The model under review builds one solid part; all positions refer to its coordinate system, in mm. Face numbers are marked on the shaded views. A direction names the side the tool comes from. Coordinates: 2 decimals unless noted, no trailing zeros. Loops run counter-clockwise (first coordinate to the right, second up) from the corner with the lowest first, then second, coordinate; pieces in that order, holes last. Notation, with made-up numbers: M 4.5,49.25 L 51.5,49.25 A28 cw 51.5,88.25 Z; hole C 5,-35.5 d2. An arc over 180 degrees is marked long. Use one line per item in the form item = value.
```python
from build123d import *

# Parameters (mm, degrees)
F3_W     = 193.8
F3_H     = 30.8805991608
F2_DEPTH = 65.3571831062
F4_R     = 6
F5_DEPTH = 5


with BuildPart() as f1:
    # F0 (on Front) → F1 (revolve)
    with BuildSketch(Plane.XZ):
        Polygon((-44.3082220923, 17.75), (-44.3082220923, 0), (345.4917779077, 0), (345.4917779077, 28), (98.3917779077, 28), (98.3917779077, 43.6), (74.3917779077, 43.6), (74.3917779077, 28), (-15.4082220923, 28), (-15.4082220923, 17.75), align=None)
    revolve(axis=Axis((24.5496360249, 0, 0), (1, 0, 0)))

    # F3 (on Front) → F2 (cut, symmetric)
    with BuildSketch(Plane.XZ):
        with Locations((233.4917779077, 15.4402995804)):
            Rectangle(F3_W, F3_H)
    extrude(amount=F2_DEPTH, both=True, mode=Mode.SUBTRACT)

    # F4 (on face) → F5 (cut)
    with BuildSketch(Plane.XY):
        with Locations((183.4917779077, 0)):
            Circle(F4_R)
        with Locations((283.4917779077, 0)):
            Circle(F4_R)
    extrude(amount=-F5_DEPTH, mode=Mode.SUBTRACT)


solid = f1.part
```
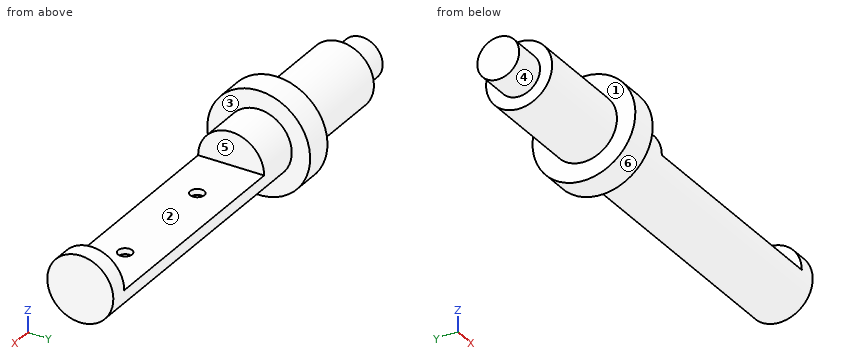
1. Insertion check: P1, Ø12, axis at x = 129, y = 14, coming from the +Z side; P2, Ø8, axis at x = 270.5, y = -20, coming from the +Z side; P3, Ø3, axis at x = 266.5, z = -27, coming from the +Y side. Each pin has a flat end and moves straight along its axis. Give the tip position at first contact, or say it passes through.
Response values:
P1 = 26.83
P2 = 0
P3 = 11.57
2. Machinability: for the marked faces 4, 5 and 6, which of the approach directions +Z, -Z, +X, -X, +Y, -Y give a long, thin tool a straight path to every point of the face, cutting with its end or side? Answer none if there is none.
Response values:
face_4 = -X
face_5 = +Z, +Y, -Y
face_6 = +X, -X
3. Add section C-C (x = 233.5). State the section outline as (y, z) points.
Response values:
outline = M -28,0 A28 ccw 28,0 Z
4. Add section A-A (y = 0). State the section outline as (x, z) points.
Response values:
outline = M -44.31,-17.75 L -15.41,-17.75 L -15.41,-28 L 74.39,-28 L 74.39,-43.6 L 98.39,-43.6 L 98.39,-28 L 345.49,-28 L 345.49,28 L 330.39,28 L 330.39,0 L 289.49,0 L 289.49,-5 L 277.49,-5 L 277.49,0 L 189.49,0 L 189.49,-5 L 177.49,-5 L 177.49,0 L 136.59,0 L 136.59,28 L 98.39,28 L 98.39,43.6 L 74.39,43.6 L 74.39,28 L -15.41,28 L -15.41,17.75 L -44.31,17.75 Z
5. Wall thickness on line 1 along X through (y, z) = (-18, 1); line 2 along X through (y, z) = (9, 13); line 3 along X through (y, z) = (26, 21): over which ranges is each line inside the solid? List them lowest first. Write a range as from..to.
Response values:
line_1 = -15.41..136.59, 330.39..345.49
line_2 = -44.31..136.59, 330.39..345.49
line_3 = 74.39..98.39
6. The part is to be moulded in two halves that separate along X. For the marked faces 1, 2 and 3, say which applies: pulls with the +X half, pulls with the -X half, needs draft (parallel to the pull), parting line crosses it, or undercut.
Response values:
face_1 = pulls with the -X half
face_2 = undercut
face_3 = pulls with the +X half
7. Add section D-D (y = 36). State the section outline as (x, z) points.
Response values:
outline = M 74.39,-24.6 L 98.39,-24.6 L 98.39,24.6 L 74.39,24.6 Z
8. Add section B-B (x = -10). State the section outline as (y, z) points, then the cut area to 3 significant figures.
Response values:
outline = C 0,0 d56
area = 2,460 mm^2
